Can you work these out from the model? Positions are in its coordinate system, mm. Give positions to 0.01 mm unless a question says otherwise; leave off trailing zeros. Write each loop counter-clockwise with the first axis right and the second up, starting at its lowest first coordinate (ties: lowest second). Pieces come first, ordered by that corner, then holes.
```python
from build123d import *

# Parameters (mm, degrees)
SKETCH1_W           = 7
SKETCH1_H           = 16
BOSS_EXTRUDE1_DEPTH = 2.9
SKETCH2_R           = 0.5
CUT_EXTRUDE1_DEPTH  = 6.8
LPATTERN1_COUNT     = 12
LPATTERN1_PITCH     = 2.54


with BuildPart() as part:
    # Sketch1 → Boss-Extrude1 (new body, symmetric)
    with BuildSketch(Plane(origin=(0, 0, 0), x_dir=(1, 0, 0), z_dir=(0, 1, 0))):
        Rectangle(SKETCH1_W, SKETCH1_H)
    extrude(amount=BOSS_EXTRUDE1_DEPTH, both=True)

    # Sketch2 → Cut-Extrude1 (cut, through all)
    with BuildSketch(Plane(origin=(0, 2.9, 0), x_dir=(1, 0, 0), z_dir=(0, 1, 0))):
        with Locations((0, 5.96)):
            Circle(SKETCH2_R)
    cut_extrude1 = extrude(amount=-CUT_EXTRUDE1_DEPTH, mode=Mode.SUBTRACT)

    # LPattern1: Cut-Extrude1 ×12
    with Locations(*[(0, 0, i * LPATTERN1_PITCH) for i in range(1, LPATTERN1_COUNT)]):
        add(cut_extrude1, mode=Mode.SUBTRACT)


solid = part.part
```
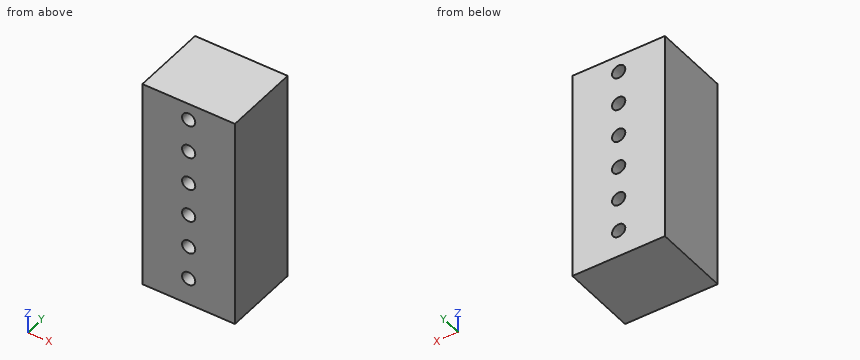
1) Suppose I cut it at C-C on y = 2.45. Write out the boundary of the cut face in (x, z).
Values follow:
outline: (-3.5, -8) - (3.5, -8) - (3.5, 8) - (-3.5, 8) - close; hole circle Ø1 at (0, -5.96); hole circle Ø1 at (0, -3.42); hole circle Ø1 at (0, -0.88); hole circle Ø1 at (0, 1.66); hole circle Ø1 at (0, 4.2); hole circle Ø1 at (0, 6.74)
2) Suppose I cut it at A-A on z = -0.88. Write out the boundary of the cut face in (x, y), plus the area to 3 significant figures.
Values follow:
outline: (-3.5, -2.9) - (-0.5, -2.9) - (-0.5, 2.9) - (-3.5, 2.9) - close; (0.5, -2.9) - (3.5, -2.9) - (3.5, 2.9) - (0.5, 2.9) - close
area: 34.8 mm2
3) Please list where these lines run through material, in increasing order: L1, parallel to X at y = -0.3, z = -3.42; L2, parallel to X at y = -2.5, z = -3.75.
Values follow:
L1: x = -3.5 to -0.5, 0.5 to 3.5
L2: x = -3.5 to -0.38, 0.38 to 3.5
4) Suppose I cut it at B-B on x = 0. Write out the boundary of the cut face in (y, z), plus the area to 3 significant figures.
Values follow:
outline: (-2.9, -8) - (2.9, -8) - (2.9, -6.46) - (-2.9, -6.46) - close; (-2.9, -5.46) - (2.9, -5.46) - (2.9, -3.92) - (-2.9, -3.92) - close; (-2.9, -2.92) - (2.9, -2.92) - (2.9, -1.38) - (-2.9, -1.38) - close; (-2.9, -0.38) - (2.9, -0.38) - (2.9, 1.16) - (-2.9, 1.16) - close; (-2.9, 2.16) - (2.9, 2.16) - (2.9, 3.7) - (-2.9, 3.7) - close; (-2.9, 4.7) - (2.9, 4.7) - (2.9, 6.24) - (-2.9, 6.24) - close; (-2.9, 7.24) - (2.9, 7.24) - (2.9, 8) - (-2.9, 8) - close
area: 58.0 mm2
